Model file for the job. Use its own axes, mm. Face numbers are marked on the shaded views. Coordinates: 2 decimals unless noted, no trailing zeros. Order: outer loops, then holes, each group sorted by start corner. A loop starts at its lowest first (then second) coordinate and runs counter-clockwise, first axis right, second up. Notation, with made-up numbers: M 55.25,55 L 105.25,55 A29 cw 105.25,77 Z; hole C 11.5,3 d10. An arc over 180 degrees is marked long. Return JSON: item names as keys, results as strings.
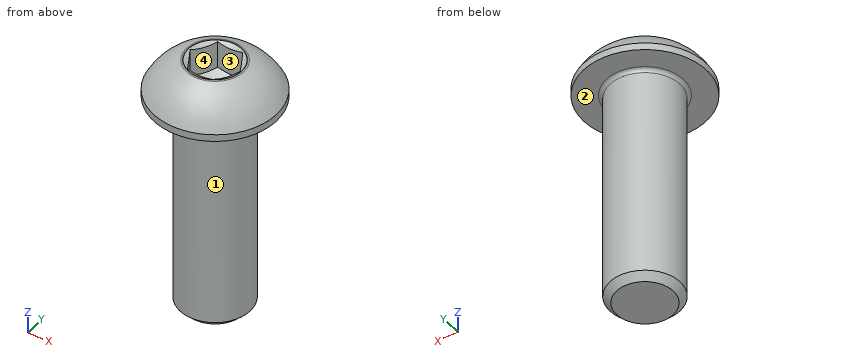
Solid Edge part; units mm, degrees
sketch "Sketch1" plane through (0, 0, 0) normal (0, -1, 0) x (1, 0, 0)
  line L0 (0, -25) -> (4, -25)
  line L1 (4, -25) -> (4, 0)
  line L2 (4, 0) -> (7, 0)
  line L3 (7, 0) -> (7, 0.8)
  arc A0 (3.1749, 4.3) -> (7, 0.8) centre (0.3366, -2.6422) cw
  line L4 (0, 4.3) -> (3.1749, 4.3)
revolve "RevolvedProtrusion1" add sketch "Sketch1" angle 360 about axis through (0, 0, 5) along (0, 0, -1)
sketch "Sketch2" plane through (0, 0, 0) normal (0, -1, 0) x (1, 0, 0)
  line L0 (0, -0.5164) -> (2.8863, 1.15)
  line L1 (2.8863, 1.15) -> (2.8863, 4.3)
  line L2 (2.8863, 4.3) -> (0, 4.3)
revolve "RevolvedCutout1" cut sketch "Sketch2" angle 360 about axis through (0, 0, 5.3) along (0, 0, -1)
sketch "Sketch3" plane through (0, 0, 0) normal (0, 0, -1) x (0, 1, 0)
  arc A0 (-2.5, 1.4425) -> (-2.5, -1.4425) centre (0, 0) ccw
  line L0 (-2.5, 1.4425) -> (-2.5, -1.4425)
extrude "Protrusion1" add sketch "Sketch3" against normal blind 4.3
pattern_circular "Pattern1" count 6 over 360 about axis through (0, 0, 0) along (0, 0, -1) of "Protrusion1"
fillet "Round_1" radius 0.375 1 edges at (-3.1749, 0, 4.3)
sketch "Sketch4" plane through (0, 0, 0) normal (0, -1, 0) x (1, 0, 0)
  line L0 (0, 2.5503) -> (3.0306, 4.3)
  line L1 (3.0306, 4.3) -> (0, 4.3)
revolve "RevolvedCutout2" cut sketch "Sketch4" angle 360 about axis through (0, 0, 5.3) along (0, 0, -1)
sketch "Sketch5" plane through (0, 0, 0) normal (0, -1, 0) x (1, 0, 0)
  line L0 (-4, 0) -> (-4.4, 0)
  arc A0 (-4.4, 0) -> (-4, -0.4) centre (-4.4, -0.4) cw
  line L1 (-4, -0.4) -> (-4, 0)
revolve "RevolvedProtrusion2" add sketch "Sketch5" angle 360 about axis through (0, 0, -1.05) along (0, 0, 1)
cosmetic_thread "Thread1"
chamfer "Chamfer1" distance 0.767 angle 45 1 edges at (-4, 0, -25)
properties material "Steel"
Item 1: Saw through at B-B (z = 0.5). Write the cut outline in (x, y).
Check result:
{"outline": "C 0,0 d14; hole C 0,0 d3.52"}
Item 2: Pull direction X, two halves, no side cores. Call the marked faces 1, 2, 3 and 4: +X half, -X half, draft (parallel to the pull), parting line (faces both ways), or undercut.
Check result:
{"face 1": "parting line", "face 2": "draft", "face 3": "undercut", "face 4": "undercut"}
Item 3: Drop flat-ended pins along their axis: pin 1 Ø8 at (y, z) = (1, -3.5) entering from +X; pin 2 Ø1.5 at (y, z) = (-1.5, -1.5) entering from -X; pin 3 Ø2 at (x, y) = (4.5, 2) entering from +Z; pin 4 Ø2.5 at (x, z) = (-0.5, 2) entering from -Y. Give the stop position or say it passes through.
Check result:
{"pin 1": "stops at x = 7", "pin 2": "stops at x = -3.93", "pin 3": "stops at z = 3.94", "pin 4": "stops at y = -7"}
Item 4: Wall check: line 1 (X direction, y = -0.25, z = -14); line 2 (Z direction, x = 5.5, y = -4); line 3 (X direction, y = 1.75, z = -19). Give the ranges that are in metal, low to high.
Check result:
{"line 1": "x = -3.99 to 3.99", "line 2": "z = 0 to 1.16", "line 3": "x = -3.6 to 3.6"}
Item 5: Saw through at A-A (z = -8.75). Write the cut outline in (x, y).
Check result:
{"outline": "C 0,0 d8"}
